Can you work these out from the model? Positions are in its coordinate system, mm. A direction names the side the tool comes from. Round coordinates to 2 decimals unless told otherwise and drop trailing zeros. Loops run counter-clockwise (first coordinate to the right, second up) from the corner with the lowest first, then second, coordinate; pieces in that order, holes last. Notation, with made-up numbers: (45, -6.5) -> (103, -6.5) arc R16 cw to (103, 10.5) -> close; hole circle Ø6 at (-4.75, 71). An arc over 180 degrees is marked (long way). Answer as a JSON object with one key per item and string values.
```python
from build123d import *

# Parameters (mm, degrees)
SKETCH1_W           = 50.8
SKETCH1_H           = 25.4
BOSS_EXTRUDE1_DEPTH = 441.450000004
SKETCH2_W           = 47.625
SKETCH2_H           = 22.225
CUT_EXTRUDE1_DEPTH  = 441.45
FILLET1_R           = 1.5875


with BuildPart() as part:
    # Sketch1 → Boss-Extrude1 (new body)
    with BuildSketch(Plane(origin=(0, 0, 0), x_dir=(0, 0, -1), z_dir=(1, 0, 0))):
        with Locations((25.4, 12.7)):
            Rectangle(SKETCH1_W, SKETCH1_H)
    extrude(amount=BOSS_EXTRUDE1_DEPTH)

    # Sketch2 → Cut-Extrude1 (cut)
    with BuildSketch(Plane.ZY):
        with Locations((-25.4, 12.7)):
            Rectangle(SKETCH2_W, SKETCH2_H)
    extrude(amount=-CUT_EXTRUDE1_DEPTH, mode=Mode.SUBTRACT)

    # Fillet1
    fillet1_edges = [part.edges().sort_by_distance(p)[0] for p in [
        (220.725000002, 25.4, 0),
        (220.725000002, 25.4, -50.8),
        (220.725000002, 0, -50.8),
        (220.725000002, 0, 0),
    ]]
    fillet(fillet1_edges, radius=FILLET1_R)


solid = part.part
```
Q1. I want a section at B-B, the plane x = 220. Write out the boundary of the cut face in (y, z) (1 decimal), then the cut area to 3 significant figures.
Determined:
{"outline": "(0, -49.2) arc R1.6 ccw to (1.6, -50.8) -> (23.8, -50.8) arc R1.6 ccw to (25.4, -49.2) -> (25.4, -1.6) arc R1.6 ccw to (23.8, 0) -> (1.6, 0) arc R1.6 ccw to (0, -1.6) -> close; hole (1.6, -49.2) -> (23.8, -49.2) -> (23.8, -1.6) -> (1.6, -1.6) -> close", "area": "230 mm²"}
Q2. I want a section at C-C, the plane y = 19.5. Write out the boundary of the cut face in (x, z), then the cut area to 3 significant figures.
Determined:
{"outline": "(0, -50.8) -> (441.45, -50.8) -> (441.45, -49.21) -> (0, -49.21) -> close; (0, -1.59) -> (441.45, -1.59) -> (441.45, 0) -> (0, 0) -> close", "area": "1,400 mm²"}
Q3. We'd pull the mould along Y, two halves only. Please class faces 1 (the flat face through (218, 0, -25)), 2 (the flat face through (218, 13, 0)), 3 (the flat face through (218, 13, -1.587)): pulls with the +Y half, pulls with the -Y half, needs draft (parallel to the pull), parting line crosses it, or undercut.
Determined:
{"face 1": "pulls with the -Y half", "face 2": "needs draft", "face 3": "undercut"}
Q4. On a 3-axis mill with a long thin cutter (end or side, diameter ignored), from which of +Z, -Z, +X, -X, +Y, -Y can I reach the whole of each face in a straight line? I mean faces 4 (the flat face through (218, 23.812, -26)), 5 (the flat face through (0, 1, -23)). Say none if no direction works.
Determined:
{"face 4": "+X, -X", "face 5": "+Z, -Z, -X, +Y, -Y"}
Q5. I'm going to push a flat-ended pin straight in: pin 1 (10 mm diameter, centred on y = 14.5, z = -23.5, fed in from -X). Where does the tip first touch, or does it pass through?
Determined:
{"pin 1": "through"}
Q6. I want a section at A-A, the plane z = -40. Write out the boundary of the cut face in (x, y).
Determined:
{"outline": "(0, 0) -> (441.45, 0) -> (441.45, 1.59) -> (0, 1.59) -> close; (0, 23.81) -> (441.45, 23.81) -> (441.45, 25.4) -> (0, 25.4) -> close"}
Q7. If I drill on L1, parallel to Y at x = 244, z = -34; L2, parallel to Z at x = 128.5, y = 23.5; L3, parallel to Z at x = 300, y = 1.5, over which ranges is the centre line in solid material (lowest first)? Write a range as [from, to].
Determined:
{"L1": "[0, 1.59], [23.81, 25.4]", "L2": "[-50.8, -49.21], [-1.59, 0]", "L3": "[-50.8, 0]"}
